Check sheet for the drawn part. Datum: minimum x, y, z corner. Units: mm. A direction names the side the tool comes from. Round coordinates to 2 decimals unless told otherwise and drop trailing zeros. Write each loop counter-clockwise with the first axis right and the second up, starting at its lowest first coordinate (ties: lowest second). Pieces come first, ordered by that corner, then holes.
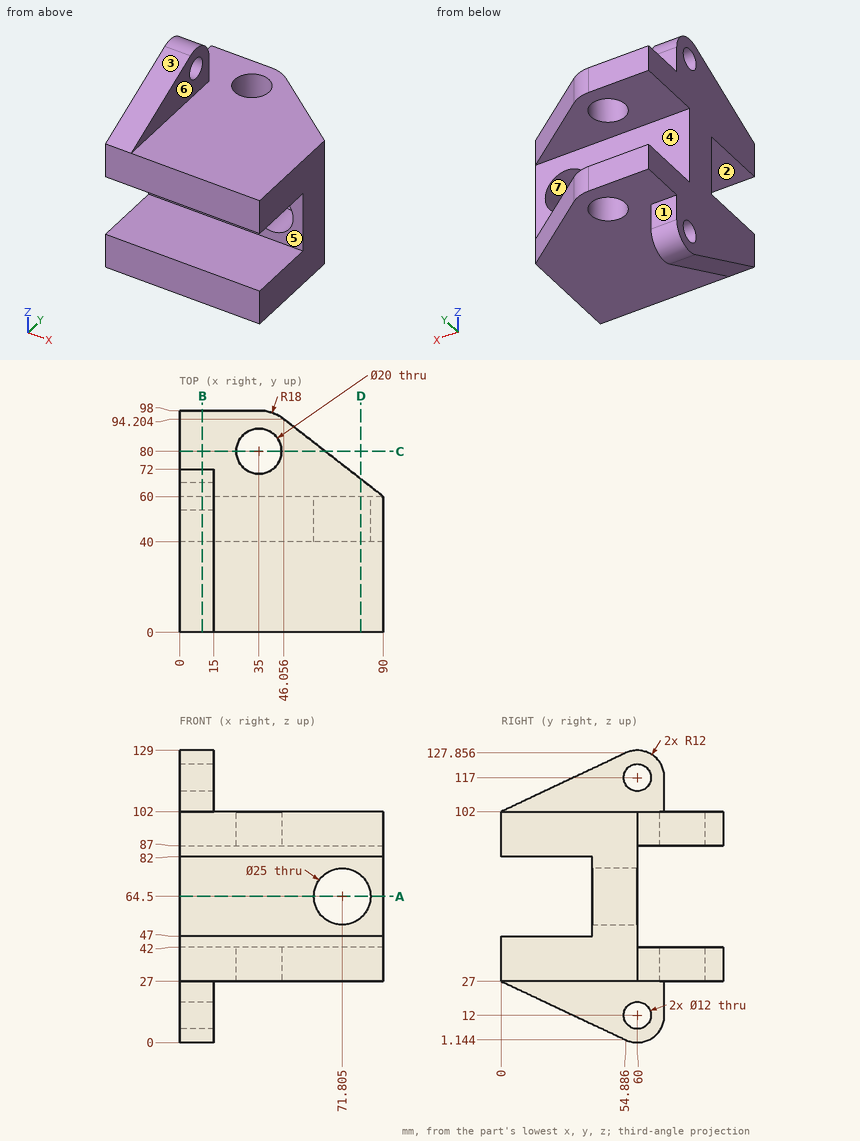
Q1. Sectioned sample at A-A (z = 64.5). Enter the section's corners in (x, y) (1 decimal).
Recorded:
outline: (0, 40) - (59.3, 40) - (59.3, 60) - (0, 60) - close; (84.3, 40) - (90, 40) - (90, 60) - (84.3, 60) - close
Q2. Sectioned sample at D-D (x = 80). Enter the section's corners in (y, z), plus the area to 3 significant figures.
Recorded:
outline: (0, 27) - (67.78, 27) - (67.78, 42) - (60, 42) - (60, 55.06) - (40, 55.06) - (40, 47) - (0, 47) - close; (0, 82) - (40, 82) - (40, 73.94) - (60, 73.94) - (60, 87) - (67.78, 87) - (67.78, 102) - (0, 102) - close
area: 2,960 mm2
Q3. Depth check by flat-ended pin: P1, Ø12, axis at x = 30.5, y = 15, coming from the -Z side; P2, Ø19, axis at y = 60, z = 117, coming from the -X side; P3, Ø10, axis at x = 21.5, z = 61, coming from the +Y side; P4, Ø19, axis at x = 42, y = 70, coming from the +Z side. Enter the tip coordinate at first touch or a pass-through.
Recorded:
P1: stops at z = 27
P2: stops at x = 0
P3: stops at y = 60
P4: stops at z = 102
Q4. Material ranges on line 1 along Z through (x, y) = (75, 18.5); line 2 along Z through (x, y) = (73, 68.5); line 3 along Y through (x, z) = (35, 94.5), recorded low to high.
Recorded:
line 1: z = 27 to 47, 82 to 102
line 2: z = 27 to 42, 87 to 102
line 3: y = 0 to 70, 90 to 98
Q5. Tool access check on the marked faces 4, 5, 6 and 7. Record the directions out of +Z, -Z, +X, -X, +Y, -Y that give a thin tool (end or side, any length) a straight path to the whole face; none if there is none.
Recorded:
face 4: +X, -X, +Y
face 5: +X, -X, -Y
face 6: +Z, +X, +Y, -Y
face 7: +Y, -Y
Q6. Sectioned sample at C-C (y = 80). Enter the section's corners in (x, z) (1 decimal), plus the area to 3 significant figures.
Recorded:
outline: (0, 27) - (25, 27) - (25, 42) - (0, 42) - close; (0, 87) - (25, 87) - (25, 102) - (0, 102) - close; (45, 27) - (64.3, 27) - (64.3, 42) - (45, 42) - close; (45, 87) - (64.3, 87) - (64.3, 102) - (45, 102) - close
area: 1,330 mm2
Q7. Sectioned sample at B-B (x = 10). Enter the section's corners in (y, z).
Recorded:
outline: (0, 27) - (54.89, 1.14) arc R12 ccw to (72, 12) - (72, 27) - (98, 27) - (98, 42) - (60, 42) - (60, 87) - (98, 87) - (98, 102) - (72, 102) - (72, 117) arc R12 ccw to (54.89, 127.86) - (0, 102) - (0, 82) - (40, 82) - (40, 47) - (0, 47) - close; hole circle Ø12 at (60, 12); hole circle Ø12 at (60, 117)
Q8. Release check for a two-part mould opening along Z. For the marked faces 1, 2 and 3 record: released by +Z, released by -Z, zero draft, split by the parting line, or undercut.
Recorded:
face 1: zero draft
face 2: undercut
face 3: released by +Z
